The listing builds one solid part. Answer for the finished solid, in the listing's coordinates (mm). A direction names the side the tool comes from. Give positions to 0.01 mm unless a question says otherwise; leave off trailing zeros. Write each loop counter-clockwise with the first axis right and the second up, starting at its lowest first coordinate (ties: lowest second). Pieces come first, ordered by that corner, then holes. Notation, with made-up numbers: (0.5, -9) - (20.5, -9) arc R23 ccw to (20.5, 6) - close; hole circle Ø5 at (84, 17). An arc over 180 degrees is marked (long way). Return JSON: item names as keys, results as strings.
Autodesk Inventor part; units mm, degrees
ref_plane "YZ Plane" through (0, 0, 0) normal (1, 0, 0) x (0, 1, 0)
ref_plane "XZ Plane" through (0, 0, 0) normal (0, 1, 0) x (-1, 0, 0)
ref_plane "XY Plane" through (0, 0, 0) normal (0, 0, 1) x (1, 0, 0)
sketch "Sketch1" plane through (0, 0, 0) normal (0, 0, 1) x (1, 0, 0)
  line L0 (0, 0) -> (187.378778, 0)
  line L1 (187.378778, -12.7) -> (0, -12.7)
  line L2 (0, 0) -> (35.7378, 0)
  line L3 (35.7378, 0) -> (35.7378, -1.5875)
  line L4 (35.7378, -1.5875) -> (36.53155, -1.5875)
  line L5 (36.53155, -1.5875) -> (36.53155, 0)
  line L6 (35.7378, -1.5875) -> (34.94405, -1.5875)
  line L7 (34.94405, -1.5875) -> (34.94405, 0)
  line L8 (36.53155, -12.7) -> (34.94405, -12.7)
  line L9 (34.94405, -12.7) -> (34.94405, -11.1125)
  line L10 (34.94405, -11.1125) -> (36.53155, -11.1125)
  line L11 (36.53155, -11.1125) -> (36.53155, -12.7)
  line L12 (187.378778, 0) -> (151.640978, 0)
sketch "Sketch3" plane through (0, 0, 0) normal (0, 0, -1) x (-1, 0, 0)
  circle A0 centre (6.35164, 38.1) radius 3.3782
  circle A1 centre (6.35164, 22.225) radius 3.3782
sketch "Sketch6" plane through (-12.7, 33.655, 109.78515) normal (0, 0, 1) x (1, 0, 0)
  line L0 (0, 0) -> (12.7, 0)
  line L1 (0, -33.655) -> (0, 0)
  line L2 (6.35, 0) -> (6.35, -11.218333)
  line L3 (6.35, -11.218333) -> (6.35, -22.445133)
  circle A0 centre (6.35, -11.218333) radius 3.3782
  circle A1 centre (6.35, -22.445133) radius 3.3782
  dimension "d29" = 11.21833
  dimension "d31" = 11.2268
  dimension "d32" = 6.7564
  dimension "d33" = 6.7564
sketch "Sketch1 outline for Plate1" plane through (0, 0, 0) normal (0, 0, 1) x (1, 0, 0)
  line L0 (0, 0) -> (-12.7, 0)
  line L1 (-12.7, 0) -> (-12.7, 44.45)
  line L2 (-12.7, 44.45) -> (0, 44.45)
  line L3 (0, 44.45) -> (0, 0)
extrude "Plate1" add sketch "Sketch1 outline for Plate1" along normal blind 3.175
sketch "Sketch2" plane through (0, -12.7, 0) normal (0, 0, 1) x (1, 0, 0)
  line L0 (35.7378, 11.1125) -> (35.7378, 12.7)
  line L1 (0, 12.7) -> (35.7378, 12.7)
  line L2 (36.53155, 12.7) -> (187.378778, 12.7)
  line L3 (35.7378, 11.1125) -> (34.94405, 11.1125)
  line L4 (34.94405, 11.1125) -> (34.94405, 12.7)
edge flange "Flange1" height 105.34015 angle 90 thickness 3.175 bend radius 1.27 thickness toward (0, -1, 0) relief straight relief width 3.175 relief depth 1.5875 edges at (-6.35, 0, 3.175) wall of the first edge with corners at (-12.7, -1.27, 4.445) (0, -1.27, 4.445) (0, -1.27, 105.34015) (-12.7, -1.27, 105.34015)
bend "Bend1"
corner "Corner1"
sketch "Sketch4" plane through (0, -12.7, 0) normal (0, 0, 1) x (1, 0, 0)
  line L0 (187.378778, 0) -> (36.53155, 0)
  line L1 (36.53155, 12.7) -> (187.378778, 12.7)
  line L2 (187.378778, 12.7) -> (140.845978, 12.7)
  line L3 (140.845978, 12.7) -> (140.845978, 11.1125)
  line L4 (140.845978, 11.1125) -> (141.639728, 11.1125)
  line L5 (141.639728, 11.1125) -> (141.639728, 12.7)
  line L6 (140.845978, 11.1125) -> (140.052228, 11.1125)
  line L7 (140.052228, 11.1125) -> (140.052228, 12.7)
  line L8 (140.845978, 0) -> (141.639728, 0)
  line L9 (141.639728, 0) -> (141.639728, 1.5875)
  line L10 (141.639728, 1.5875) -> (140.052228, 1.5875)
  line L11 (140.052228, 1.5875) -> (140.052228, 0)
  dimension "d15" = 1.5875
extrude "Cut1" cut sketch "Sketch3" against normal blind 3.175
sketch "Sketch5" plane through (0, -12.7, 0) normal (0, 0, 1) x (1, 0, 0)
  line L0 (140.845978, 12.7) -> (140.845978, 11.1125)
  line L1 (140.845978, 12.7) -> (187.378778, 12.7)
  line L2 (140.845978, 11.1125) -> (141.639728, 11.1125)
  line L3 (141.639728, 11.1125) -> (141.639728, 12.7)
edge flange "Flange2" height 38.1 angle 90 thickness 3.175 bend radius 1.27 thickness toward (0, 0, 1) relief straight relief width 3.175 relief depth 1.5875 edges at (-6.35, -1.27, 105.34015) wall of the first edge with corners at (-12.7, 0, 106.61015) (0, 0, 106.61015) (0, 33.655, 106.61015) (-12.7, 33.655, 106.61015)
bend "Bend2"
corner "Corner2"
extrude "Cut3" cut sketch "Sketch6" against normal blind 3.175
equation "\"d3\" = BendReliefWidth"
equation "\"d4\" = BendReliefDepth"
equation "\"d5\" = MinimumRemnant"
equation "\"d6\" = BendRadius"
equation "\"d10\" = CornerReliefSize"
equation "\"d11\" = GapSize"
equation "\"d12\" = JacobiRadiusSize"
equation "\"d19\" = BendReliefWidth"
equation "\"d20\" = BendReliefDepth"
equation "\"d21\" = MinimumRemnant"
equation "\"d22\" = BendRadius"
equation "\"d26\" = CornerReliefSize"
equation "\"d27\" = GapSize"
equation "\"d28\" = JacobiRadiusSize"
equation "\"BendRadius\" = Thickness"
equation "\"BendReliefWidth\" = Thickness"
equation "\"BendReliefDepth\" = 0.5 * Thickness"
equation "\"CornerReliefSize\" = 4 * Thickness"
equation "\"MinimumRemnant\" = 2 * Thickness"
equation "\"TransitionRadius\" = BendRadius"
equation "\"JacobiRadiusSize\" = Thickness"
equation "\"GapSize\" = Thickness"
equation "\"d2\" = BendRadius"
equation "\"d6\" = Thickness"
equation "\"d16\" = Thickness"
properties part number "bottom pulley mount"
Item 1: Flat-ended cylindrical pins translate along their axes: P1, Ø2.5, axis at x = -8.5, z = 108, coming from the +Y side (3 decimals); P2, Ø5.5, axis at x = -6.35, y = 22.44, coming from the -Z side. Find the tip coordinate at first contact, or state that the pin passes through.
Answer below:
{"P1": "stops at y = 33.655", "P2": "passes through"}
Item 2: A cutting plane is placed at C-C on y = 10. Determine the outline of the cut face in (x, z) (3 decimals), then the cut area to 3 significant figures.
Answer below:
{"outline": "(-12.7, 0) - (0, 0) - (0, 3.175) - (-12.7, 3.175) - close; (-12.7, 106.61) - (-9.504, 106.61) - (-9.504, 109.785) - (-12.7, 109.785) - close; (-3.196, 106.61) - (0, 106.61) - (0, 109.785) - (-3.196, 109.785) - close", "area": "60.6 mm²"}
Item 3: The mould has two halves that part along Y. Classify faces 6 (the face through (-6, 18, 0)), 7 (the face through (-6, -1.27, 54)), 8 (the face through (-3.229, 9.916, 108.22)): +Y half, -Y half, draft (parallel to the pull), parting line (faces both ways), or undercut.
Answer below:
{"face 6": "draft", "face 7": "+Y half", "face 8": "undercut"}
Item 4: Consider L1, parallel to Y at x = -6.35, z = 108.15 (3 decimals); L2, parallel to Z at x = -0.75, y = 31.5 (3 decimals); L3, parallel to Y at x = -6.35, z = 109.1 (3 decimals). Determine where each line is inside the solid, lowest interval first.
Answer below:
{"L1": "y = -3.444 to 7.832, 14.588 to 19.058, 25.815 to 33.655", "L2": "z = 0 to 3.175, 106.61 to 109.785", "L3": "y = -2.371 to 7.832, 14.588 to 19.058, 25.815 to 33.655"}
Item 5: A cutting plane is placed at A-A on y = 38.1. Determine the outline of the cut face in (x, z) (3 decimals), then the cut area to 3 significant figures.
Answer below:
{"outline": "(-12.7, 0) - (-9.73, 0) - (-9.73, 3.175) - (-12.7, 3.175) - close; (-2.973, 0) - (0, 0) - (0, 3.175) - (-2.973, 3.175) - close", "area": "18.9 mm²"}
Item 6: For faces 1 (the face through (-6.261, -3.108, 108.518)), 2 (the face through (-5.619, 18.927, 1.565)), 3 (the face through (-4.79, 19.44, 108.22)), 4 (the face through (-6, 33.655, 108)), 5 (the face through (-6, 17, 106.61)), determine the directions among +Z, -Z, +X, -X, +Y, -Y from which every point of the face is accessible in a straight line to the end or side of a thin tool.
Answer below:
{"face 1": "+Z, +X, -X, -Y", "face 2": "-Z", "face 3": "+Z", "face 4": "+Z, +X, -X, +Y", "face 5": "+X, -X, +Y"}
Item 7: A cutting plane is placed at D-D on x = -11.5. Determine the outline of the cut face in (y, z) (3 decimals), then the cut area to 3 significant figures.
Answer below:
{"outline": "(-4.445, 4.445) arc R4.445 ccw to (0, 0) - (44.45, 0) - (44.45, 3.175) - (0, 3.175) arc R1.27 cw to (-1.27, 4.445) - (-1.27, 105.34) arc R1.27 cw to (0, 106.61) - (33.655, 106.61) - (33.655, 109.785) - (0, 109.785) arc R4.445 ccw to (-4.445, 105.34) - close", "area": "597 mm²"}
Item 8: A cutting plane is placed at B-B on x = -6.35. Determine the outline of the cut face in (y, z) (3 decimals), then the cut area to 3 significant figures.
Answer below:
{"outline": "(-4.445, 4.445) arc R4.445 ccw to (0, 0) - (18.847, 0) - (18.847, 3.175) - (0, 3.175) arc R1.27 cw to (-1.27, 4.445) - (-1.27, 105.34) arc R1.27 cw to (0, 106.61) - (7.832, 106.61) - (7.832, 109.785) - (0, 109.785) arc R4.445 ccw to (-4.445, 105.34) - close; (14.588, 106.61) - (19.058, 106.61) - (19.058, 109.785) - (14.588, 109.785) - close; (25.603, 0) - (34.722, 0) - (34.722, 3.175) - (25.603, 3.175) - close; (25.815, 106.61) - (33.655, 106.61) - (33.655, 109.785) - (25.815, 109.785) - close; (41.478, 0) - (44.45, 0) - (44.45, 3.175) - (41.478, 3.175) - close", "area": "511 mm²"}
